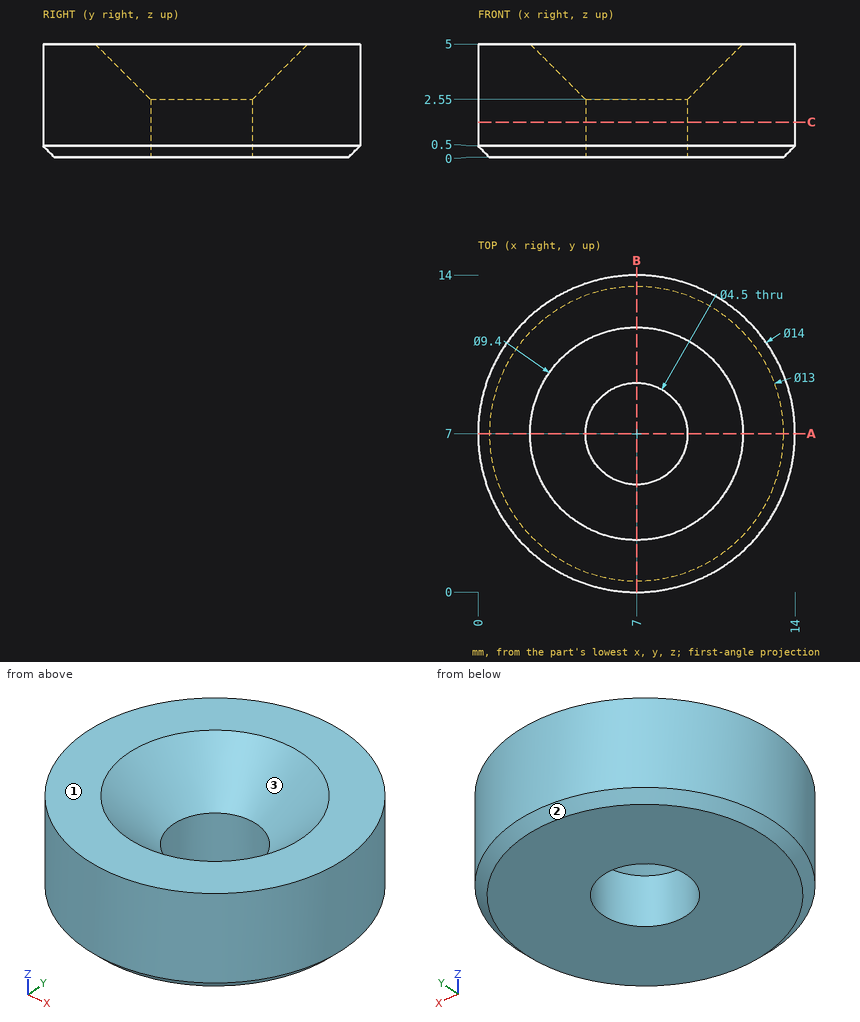
Print and shaded views of the part. All mm, measured from the part's lowest x, y and z. Round coordinates to 2 decimals unless told otherwise and drop trailing zeros. Write each loop counter-clockwise with the first axis right and the second up, starting at its lowest first coordinate (ties: lowest second). Pieces come first, ordered by that corner, then holes. Notation, with made-up numbers: (-24.75, 64) - (14.25, 64) arc R16 ccw to (14.25, 82) - close; hole circle Ø1 at (-24, 66.25). An arc over 180 degrees is marked (long way). Use CSV: the item, a comma, the result in double quotes. Start each with the question number.
Item 1: Pin check, flat tips, straight feed: P1, Ø4, axis at x = 7, y = 7, coming from the +Z side; P2, Ø1, axis at x = 5.5, z = 2, coming from the +Y side. Stop position of each tip, or through.
Item 2: Band-saw the part on C-C (z = 1.55). Write the cut outline in (x, y).
Item 3: Two-plate mould, pull along X, no slides. Class the marked faces 1, 2 and 3: released by +X, released by -X, zero draft, split by the parting line, or undercut.
Item 4: Band-saw the part on A-A (y = 7). Write the cut outline in (x, z), and give its area (3 significant figures).
Item 5: Drill centre lines: L1, parallel to Y at x = 7, z = 1.7; L2, parallel to X at y = 7.25, z = 4.2; L3, parallel to Y at x = 6.75, z = 3.2. Where is each one in solid material? Low to high. Write a range as [from, to].
Checked values:
1,P1,"passes through"
1,P2,"stops at y = 13.93"
2,outline,"circle Ø14 at (7, 7); hole circle Ø4.5 at (7, 7)"
3,face 1,"zero draft"
3,face 2,"split by the parting line"
3,face 3,"undercut"
4,outline,"(0, 0.5) - (0.5, 0) - (4.75, 0) - (4.75, 2.55) - (2.3, 5) - (0, 5) - close; (9.25, 0) - (13.5, 0) - (14, 0.5) - (14, 5) - (11.7, 5) - (9.25, 2.55) - close"
4,area,"41.2 mm²"
5,L1,"y = [0, 4.75], [9.25, 14]"
5,L2,"x = [0, 3.11], [10.89, 14]"
5,L3,"y = [0, 4.11], [9.89, 14]"
